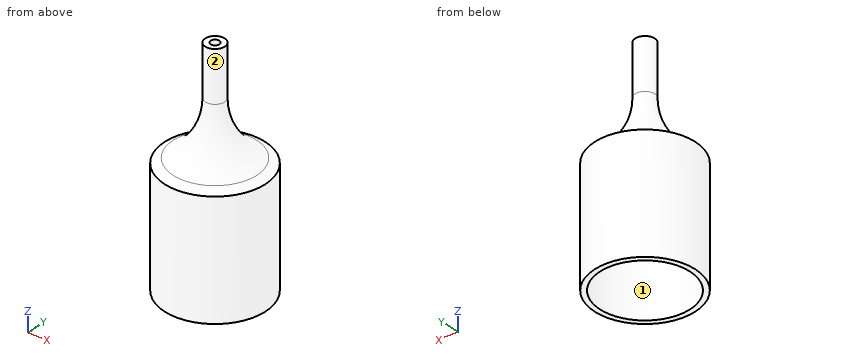
```python
from build123d import *


with BuildPart() as f2:
    # F0 (on Front) → F2 (revolve)
    with BuildSketch(Plane.XZ):
        with BuildLine():
            Line((-28.4, 0), (-25.4, 0))
            Line((-25.4, 0), (-25.4, 63.5))
            Line((-25.4, 63.5), (-22.121717, 65.318087))
            ThreePointArc((-22.121717, 65.318087), (-7.769887, 79.303451), (-2.5, 98.637197))
            Line((-2.5, 98.637197), (-2.5, 127))
            Line((-2.5, 127), (-5.5, 127))
            Line((-5.5, 127), (-5.5, 98.637197))
            ThreePointArc((-5.5, 98.637197), (-10.354936, 80.825794), (-23.5767, 67.941639))
            Line((-23.5767, 67.941639), (-28.4, 65.266708))
            Line((-28.4, 65.266708), (-28.4, 0))
        make_face()
    revolve(axis=Axis((0, 0, 64.849392), (0, 0, 1)))


solid = f2.part
```
Design review of the part built by this model. Coordinates are the model's own, in mm. Face numbers are marked on the shaded views. Give positions to 0.01 mm unless a question says otherwise; leave off trailing zeros. Write each loop counter-clockwise with the first axis right and the second up, starting at its lowest first coordinate (ties: lowest second). Pieces come first, ordered by that corner, then holes. Notation, with made-up numbers: (-5.5, 53) - (26.5, 53) arc R8 ccw to (26.5, 60) - close; hole circle Ø5 at (79, 77). An arc over 180 degrees is marked (long way). Return JSON: item names as keys, results as strings. Group by question number.
(1) We need section C-C, the plane z = 28. Give the boundary of the cut face in (x, y), then the cut area to 3 significant figures.
(2) To check wall thickness, follow probe 1 along Y at (x, z) = (0, 118.25); probe 2 along Y at (x, z) = (0, 14). State the ranges of each line that lie inside material, in increasing order.
(3) We need section D-D, the plane z = 76. Give the boundary of the cut face in (x, y), then the cut area to 3 significant figures.
(4) We need section A-A, the plane x = 0. Give the boundary of the cut face in (y, z).
(5) Mouldability with a two-part tool opening along X and no side actions: class the marked faces 1 and 2 as +X half, -X half, draft (parallel to the pull), parting line (faces both ways), or undercut.
(6) Insertion check: pin 1 (3 mm diameter, centred on x = -7.5, z = 78.5, fed in from -Y); pin 2 (1 mm diameter, centred on y = 0.5, z = 82.5, fed in from +X); pin 3 (1.5 mm diameter, centred on x = -14.5, y = 4, fed in from +Z). Each pin has a flat end and moves straight along its axis. Give the tip position at first contact, or say it passes through.
Reported:
{
 "1": {"outline": "circle Ø56.8 at (0, 0); hole circle Ø50.8 at (0, 0)", "area": "507 mm2"},
 "2": {"probe 1": "y = -5.5 to -2.5, 2.5 to 5.5", "probe 2": "y = -28.4 to -25.4, 25.4 to 28.4"},
 "3": {"outline": "circle Ø27.55 at (0, 0); hole circle Ø19.91 at (0, 0)", "area": "285 mm2"},
 "4": {"outline": "(-28.4, 0) - (-25.4, 0) - (-25.4, 63.5) - (-22.12, 65.32) arc R38.1 ccw to (-2.5, 98.64) - (-2.5, 127) - (-5.5, 127) - (-5.5, 98.64) arc R35.1 cw to (-23.58, 67.94) - (-28.4, 65.27) - close; (2.5, 98.64) arc R38.1 ccw to (22.12, 65.32) - (25.4, 63.5) - (25.4, 0) - (28.4, 0) - (28.4, 65.27) - (23.58, 67.94) arc R35.1 cw to (5.5, 98.64) - (5.5, 127) - (2.5, 127) - close"},
 "5": {"face 1": "undercut", "face 2": "parting line"},
 "6": {"pin 1": "stops at y = -10.89", "pin 2": "stops at x = 9.68", "pin 3": "stops at z = 75.4"}
}
